from build123d import *

# Parameters (mm, degrees)
SKETCH002_R  = 5
PAD002_DEPTH = 7
SKETCH_R     = 1.15
POCKET_DEPTH = 5
SKETCH003_R  = 1.3
PAD_DEPTH    = 3


with BuildPart() as part:
    # Sketch002 → Pad002 (new body)
    with BuildSketch(Plane(origin=(0, 0, 0), x_dir=(-1, 0, 0), z_dir=(0, 0, 1))):
        Circle(SKETCH002_R)
        with BuildLine():
            ThreePointArc((2.15, 1.549193), (-2.65, 0), (2.15, -1.549193))
            Line((2.15, 1.549193), (2.15, -1.549193))
        make_face(mode=Mode.SUBTRACT)
    extrude(amount=-PAD002_DEPTH)

    # Sketch → Pocket (cut)
    with BuildSketch(Plane(origin=(0, 0, -3.5), x_dir=(0, 1, 0), z_dir=(1, 0, 0))):
        Circle(SKETCH_R)
    extrude(amount=-POCKET_DEPTH, mode=Mode.SUBTRACT)

    # Sketch003 → Pad (join)
    with BuildSketch(Plane.XY):
        with BuildLine():
            Line((-41, 5), (-8.5, 5))
            ThreePointArc((-8.5, 5), (-6.025126, 6.025126), (-5, 8.5))
            Line((-5, 8.5), (-5, 41))
            ThreePointArc((-1, 45), (-3.828427, 43.828427), (-5, 41))
            Line((-1, 45), (1, 45))
            ThreePointArc((5, 41), (3.828427, 43.828427), (1, 45))
            Line((5, 41), (5, 8.5))
            ThreePointArc((5, 8.5), (6.025126, 6.025126), (8.5, 5))
            Line((8.5, 5), (41, 5))
            ThreePointArc((45, 1), (43.828427, 3.828427), (41, 5))
            Line((45, 1), (45, -1))
            ThreePointArc((41, -5), (43.828427, -3.828427), (45, -1))
            Line((41, -5), (8.5, -5))
            ThreePointArc((8.5, -5), (6.025126, -6.025126), (5, -8.5))
            Line((5, -8.5), (5, -41))
            ThreePointArc((1, -45), (3.828427, -43.828427), (5, -41))
            Line((1, -45), (-1, -45))
            ThreePointArc((-5, -41), (-3.828427, -43.828427), (-1, -45))
            Line((-5, -41), (-5, -8.5))
            ThreePointArc((-5, -8.5), (-6.025126, -6.025126), (-8.5, -5))
            Line((-8.5, -5), (-41, -5))
            ThreePointArc((-45, -1), (-43.828427, -3.828427), (-41, -5))
            Line((-45, -1), (-45, 1))
            ThreePointArc((-41, 5), (-43.828427, 3.828427), (-45, 1))
        make_face()
        with Locations((39, 0)):
            Circle(SKETCH003_R, mode=Mode.SUBTRACT)
        with Locations((-39, 0)):
            Circle(SKETCH003_R, mode=Mode.SUBTRACT)
        with Locations((0, 39)):
            Circle(SKETCH003_R, mode=Mode.SUBTRACT)
        with Locations((0, -39)):
            Circle(SKETCH003_R, mode=Mode.SUBTRACT)
    extrude(amount=PAD_DEPTH)


solid = part.part
Can you work these out from the model? Positions are in its coordinate system, mm. A direction names the side the tool comes from. Give positions to 0.01 mm unless a question says otherwise; leave off trailing zeros. Write each loop counter-clockwise with the first axis right and the second up, starting at its lowest first coordinate (ties: lowest second). Pieces come first, ordered by that corner, then holes. Notation, with made-up numbers: (54, -0.75) -> (107, -0.75) arc R22 ccw to (107, 29.25) -> close; hole circle Ø2 at (12.25, 34.25). An arc over 180 degrees is marked (long way). Answer as a JSON object with one key per item and string values. Group by question number.
Item 1: Suppose I cut it at C-C (z = -3.5). Please give me the cut outline in (x, y).
Item 2: We'd pull the mould along Y, two halves only. Please class faces 1 (the face through (-6.05, 6, 1.48)), 2 (the face through (4, 4, 0)), 3 (the face through (-40.3, 0.06, 1.48)): +Y half, -Y half, draft (parallel to the pull), parting line (faces both ways), or undercut.
Item 3: Please list where these lines run through material, in increasing order: line 1 (Y direction, x = 0, z = 1.45); line 2 (Y direction, x = 39, z = 1.9); line 3 (Y direction, x = -4.25, z = -3.5). Write a range as [from, to].
Item 4: Suppose I cut it at A-A (y = -39). Please give me the cut outline in (x, z), plus the area to 3 significant figures.
Item 5: Suppose I cut it at D-D (y = -11). Please give me the cut outline in (x, z), plus the area to 3 significant figures.
Item 6: For faces 4 (the face through (-25, 5, 1)), 5 (the face through (25, 5, 1)), 6 (the face through (25, -5, 1)), which set-ups out of +Z, -Z, +X, -X, +Y, -Y let a thin tool reach every point of the face, with its end or its side?
Item 7: I'm going to push flat-ended pins straight in: P1, Ø0.9, axis at y = 0.5, z = -5, coming from the +X side; P2, Ø4, axis at x = 34, z = -1, coming from the +Y side; P3, Ø3.5, axis at x = 29.5, z = 2, coming from the -Y side; P4, Ø2, axis at x = 39, y = 0, coming from the -Z side. Where does each tip first touch, or does it pass through?
Findings:
{
 "1": {"outline": "(-4.87, -1.15) arc R5 ccw (long way) to (-4.87, 1.15) -> (-2.15, 1.15) -> (-2.15, 1.55) arc R2.65 cw (long way) to (-2.15, -1.55) -> (-2.15, -1.15) -> close"},
 "2": {"face 1": "+Y half", "face 2": "draft", "face 3": "undercut"},
 "3": {"line 1": "y = [-45, -40.3], [-37.7, 37.7], [40.3, 45]", "line 2": "y = [-5, -1.3], [1.3, 5]", "line 3": "y = [-2.63, -1.15], [1.15, 2.63]"},
 "4": {"outline": "(-5, 0) -> (-1.3, 0) -> (-1.3, 3) -> (-5, 3) -> close; (1.3, 0) -> (5, 0) -> (5, 3) -> (1.3, 3) -> close", "area": "22.2 mm²"},
 "5": {"outline": "(-5, 0) -> (5, 0) -> (5, 3) -> (-5, 3) -> close", "area": "30.0 mm²"},
 "6": {"face 4": "+Z, -Z, -X, +Y", "face 5": "+Z, -Z, +X, +Y", "face 6": "+Z, -Z, +X, -Y"},
 "7": {"P1": "stops at x = 5", "P2": "stops at y = 5", "P3": "stops at y = -5", "P4": "passes through"}
}
